Work out the finished part from the listing and answer in its coordinate system (mm). A direction names the side the tool comes from. Round coordinates to 2 decimals unless told otherwise and drop trailing zeros. Order: outer loops, then holes, each group sorted by start corner. A loop starts at its lowest first (then second) coordinate and runs counter-clockwise, first axis right, second up. Notation, with made-up numbers: (30.25, 17.25) - (87.25, 17.25) arc R21 cw to (87.25, 32.25) - close; hole circle Ø10 at (89.5, 86). An arc over 180 degrees is marked (long way). Use one line per item in the form item = value. Start each with the question number.
Q1. Find the intervals of material crossed by line 1 (Z direction, x = 159.5, y = 19) (3 decimals); line 2 (Y direction, x = 178, z = -38.1) (1 decimal); line 3 (X direction, y = 46, z = -10) (3 decimals), in increasing order. Write a range as [from, to].
Q2. Which of the six approach directions +Z, -Z, +X, -X, +Y, -Y give full straight-line access (tool end or side, diameter ignored) to faces 5 (the flat face through (99, 31.75, -14)), 6 (the flat face through (9, 73.025, -38)), 7 (the flat face through (97, 15.875, -54)), 8 (the flat face through (97, 22.225, -73))?
Q3. Given P1, Ø5.5, axis at x = 20.5, z = -39, coming from the -Y side (3 decimals); P2, Ø3.5, axis at y = 75, z = -40.5, coming from the -X side; P3, Ø23, axis at x = 109, z = -66.5, coming from the +Y side, each flat-ended and moving along its own axis, determine where each tip first touches the part or whether it passes through.
Q4. For a pull along Y with two mould halves and no side action, classify faces 1 (the flat face through (94, 5, -76.2)), 2 (the cylindrical face through (176.413, 61.768, -14.752)), 3 (the flat face through (97, 9.525, -73)), 4 (the flat face through (97, 16, -6.35)) as +Y half, -Y half, draft (parallel to the pull), parting line (faces both ways), or undercut.
Q5. The part is cut by section C-C on x = 142.5. Determine the outline of the cut face in (y, z) (3 decimals), plus the area to 3 significant figures.
Q6. The part is cut by section B-B on z = -38.1. Determine the outline of the cut face in (x, y) (1 decimal).
Q7. The part is cut by section A-A on y = 50.8. Determine the outline of the cut face in (x, z) (1 decimal).
from build123d import *

# Parameters (mm, degrees)
EXTRUDE1_DEPTH = 76.2
EXTRUDE2_DEPTH = 28.575
SKETCH4_R      = 7.9375
EXTRUDE3_DEPTH = 76.2
EXTRUDE4_DEPTH = 219.867836833
SKETCH6_W      = 12.7
SKETCH6_H      = 12.7
EXTRUDE5_DEPTH = 219.867836833


with BuildPart() as part:
    # Sketch2 → Extrude1 (new body)
    with BuildSketch(Plane.XY):
        Polygon((17.4625, 76.2), (17.4625, 73.025), (0, 73.025), (0, 0), (190.5, 0), (190.5, 76.2), (161.925, 76.2), (161.925, 31.75), (34.925, 31.75), (34.925, 76.2), align=None)
    extrude(amount=-EXTRUDE1_DEPTH)

    # Sketch3 → Extrude2 (cut)
    with BuildSketch(Plane(origin=(190.5, 0, 0), x_dir=(0, 0, -1), z_dir=(1, 0, 0))):
        with BuildLine():
            Line((0, 55.5625), (0, 76.2))
            Line((0, 76.2), (20.6375, 76.2))
            ThreePointArc((20.6375, 76.2), (14.592916197, 61.607083803), (0, 55.5625))
        make_face()
        with BuildLine():
            Line((76.2, 76.2), (55.5625, 76.2))
            ThreePointArc((55.5625, 76.2), (61.607083803, 61.607083803), (76.2, 55.5625))
            Line((76.2, 55.5625), (76.2, 76.2))
        make_face()
    extrude(amount=-EXTRUDE2_DEPTH, mode=Mode.SUBTRACT)

    # Sketch4 → Extrude3 (cut)
    with BuildSketch(Plane(origin=(190.5, 0, 0), x_dir=(0, 0, -1), z_dir=(1, 0, 0))):
        with Locations((38.1, 50.8)):
            Circle(SKETCH4_R)
    extrude(amount=-EXTRUDE3_DEPTH, mode=Mode.SUBTRACT)

    # Sketch5 → Extrude4 (cut, through all)
    with BuildSketch(Plane(origin=(190.5, 0, 0), x_dir=(0, 0, -1), z_dir=(1, 0, 0))):
        Polygon((15.875, 15.875), (28.575, 15.875), (28.575, 34.925), (47.625, 34.925), (47.625, 15.875), (60.325, 15.875), (60.325, 0), (15.875, 0), align=None)
    extrude(amount=-EXTRUDE4_DEPTH, mode=Mode.SUBTRACT)

    # Sketch6 → Extrude5 (cut, through all)
    with BuildSketch(Plane(origin=(190.5, 0, 0), x_dir=(0, 0, -1), z_dir=(1, 0, 0))):
        with Locations((0, 15.875)):
            Rectangle(SKETCH6_W, SKETCH6_H)
        with Locations((76.2, 15.875)):
            Rectangle(SKETCH6_W, SKETCH6_H)
    extrude(amount=-EXTRUDE5_DEPTH, mode=Mode.SUBTRACT)


solid = part.part
Found:
q1.line_1 = [-69.85, -47.625], [-28.575, -6.35]
q1.line_2 = [34.9, 42.9], [58.7, 76.2]
q1.line_3 = [0, 34.925], [161.925, 190.5]
q2.face_5 = +Z, -Z, +Y
q2.face_6 = +Z, -Z, -X, +Y
q2.face_7 = +X, -X, -Y
q2.face_8 = -Z, +X, -X
q3.P1 = 34.925
q3.P2 = 17.46
q3.P3 = 31.75
q4.face_1 = draft
q4.face_2 = +Y half
q4.face_3 = undercut
q4.face_4 = undercut
q5.outline = (0, -76.2) - (9.525, -76.2) - (9.525, -69.85) - (22.225, -69.85) - (22.225, -76.2) - (31.75, -76.2) - (31.75, -47.625) - (15.875, -47.625) - (15.875, -60.325) - (0, -60.325) - close; (0, -15.875) - (15.875, -15.875) - (15.875, -28.575) - (31.75, -28.575) - (31.75, 0) - (22.225, 0) - (22.225, -6.35) - (9.525, -6.35) - (9.525, 0) - (0, 0) - close
q5.area = 1,250 mm²
q6.outline = (0, 34.9) - (34.9, 34.9) - (34.9, 76.2) - (17.5, 76.2) - (17.5, 73) - (0, 73) - close; (161.9, 34.9) - (190.5, 34.9) - (190.5, 42.9) - (161.9, 42.9) - close; (161.9, 58.7) - (190.5, 58.7) - (190.5, 76.2) - (161.9, 76.2) - close
q7.outline = (0, -76.2) - (34.9, -76.2) - (34.9, 0) - (0, 0) - close; (161.9, -76.2) - (190.5, -76.2) - (190.5, -46) - (161.9, -46) - close; (161.9, -30.2) - (190.5, -30.2) - (190.5, 0) - (161.9, 0) - close
